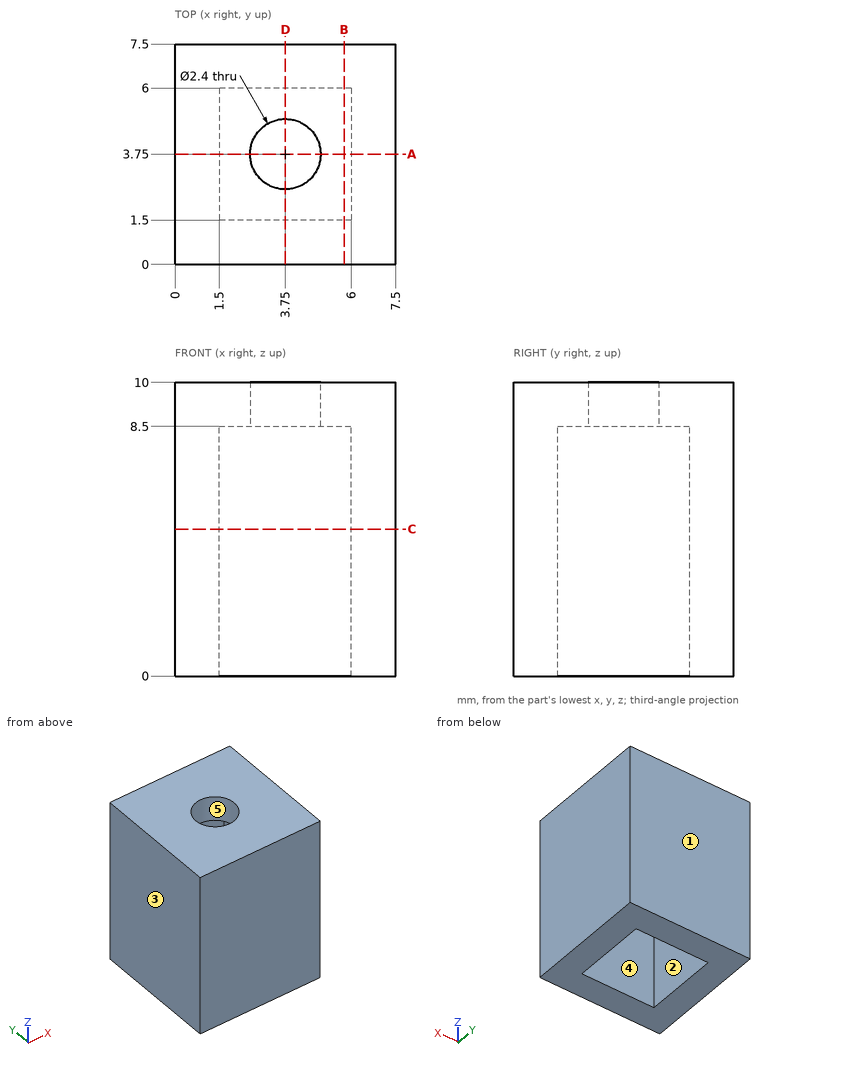
Print and shaded views of the part. All mm, measured from the part's lowest x, y and z. A direction names the side the tool comes from. Give positions to 0.01 mm unless a question says otherwise; leave off trailing zeros. Write each loop counter-clockwise with the first axis right and the second up, starting at its lowest first coordinate (ties: lowest second). Pieces come first, ordered by that corner, then holes. Notation, with made-up numbers: (-7, -22.75) -> (-2, -22.75) arc R10 cw to (-2, -6.75) -> close; hole circle Ø5 at (-10, 18). An arc over 180 degrees is marked (long way). Write item = value, one per line.
(1) Tool access for the marked faces 4 and 5: list every direction of +Z, -Z, +X, -X, +Y, -Y with a clear straight run to the whole face (end or side of a thin tool).
Determined:
face_4 = -Z
face_5 = +Z, -Z
(2) Flat gauge pin, fed straight in: P1, Ø3, axis at x = 3.5, y = 4, coming from the -Z side. Where does the tip first touch, or does it go through?
Determined:
P1 = 8.5
(3) Probe line 1 along X through (y, z) = (1.75, 7.25); line 2 along X through (y, z) = (3.75, 8.9). List the from-to ranges inside material, lowest first.
Determined:
line_1 = 0 to 1.5, 6 to 7.5
line_2 = 0 to 2.55, 4.95 to 7.5
(4) Slice it at A-A, the plane y = 3.75. Give the cut face in (x, z), then the cut area to 4 significant figures.
Determined:
outline = (0, 0) -> (1.5, 0) -> (1.5, 8.5) -> (2.55, 8.5) -> (2.55, 10) -> (0, 10) -> close; (4.95, 8.5) -> (6, 8.5) -> (6, 0) -> (7.5, 0) -> (7.5, 10) -> (4.95, 10) -> close
area = 33.15 mm2
(5) Slice it at C-C, the plane z = 5. Give the cut face in (x, y).
Determined:
outline = (0, 0) -> (7.5, 0) -> (7.5, 7.5) -> (0, 7.5) -> close; hole (1.5, 1.5) -> (6, 1.5) -> (6, 6) -> (1.5, 6) -> close
(6) Slice it at B-B, the plane x = 5.75. Give the cut face in (y, z).
Determined:
outline = (0, 0) -> (1.5, 0) -> (1.5, 8.5) -> (6, 8.5) -> (6, 0) -> (7.5, 0) -> (7.5, 10) -> (0, 10) -> close
(7) Mould opens along X. For the marked faces 1, 2 and 3 say: released by +X, released by -X, zero draft, split by the parting line, or undercut.
Determined:
face_1 = zero draft
face_2 = undercut
face_3 = released by -X
